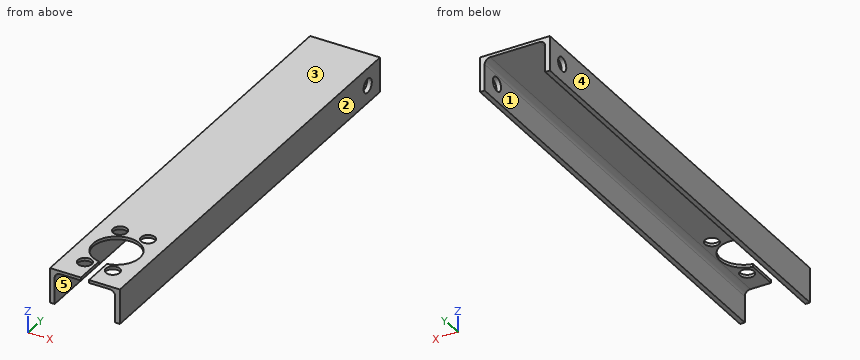
```python
from build123d import *

# Parameters (mm, degrees)
F1_DEPTH = 635
F3_DEPTH = 4.2
F4_R     = 10
F5_DEPTH = 4.2
F6_R     = 10
F7_DEPTH = 100


with BuildPart() as f1:
    # F0 (on Front) → F1 (new body)
    with BuildSketch(Plane.XZ):
        with BuildLine():
            Line((50, 0), (0, 0))
            Line((0, 0), (-50, 0))
            Line((-50, 0), (-50, -50))
            Line((-50, -50), (-43.3, -50))
            Line((-43.3, -50), (-43.3, -12.2))
            ThreePointArc((-43.3, -12.2), (-40.956854, -6.543146), (-35.3, -4.2))
            Line((-35.3, -4.2), (0, -4.2))
            Line((0, -4.2), (35.3, -4.2))
            ThreePointArc((35.3, -4.2), (40.956854, -6.543146), (43.3, -12.2))
            Line((43.3, -12.2), (43.3, -50))
            Line((43.3, -50), (50, -50))
            Line((50, -50), (50, 0))
        make_face()
    extrude(amount=-F1_DEPTH)

    # F2 (on face) → F3 (cut, through all)
    with BuildSketch(Plane.XY):
        with BuildLine():
            Line((5.75, 0), (5.75, 43.997159))
            ThreePointArc((5.75, 43.997159), (0, 110.5), (-5.75, 43.997159))
            Line((-5.75, 43.997159), (-5.75, 0))
            Line((-5.75, 0), (5.75, 0))
        make_face()
    extrude(amount=-F3_DEPTH, mode=Mode.SUBTRACT)

    # F4 (on face) → F5 (cut, through all)
    with BuildSketch(Plane.XY):
        with Locations((-20, 34)):
            Circle(F4_R)
        with Locations((-20, 120)):
            Circle(F4_R)
        with Locations((20, 34)):
            Circle(F4_R)
        with Locations((20, 120)):
            Circle(F4_R)
    extrude(amount=-F5_DEPTH, mode=Mode.SUBTRACT)

    # F6 (on face) → F7 (cut, through all)
    with BuildSketch(Plane(origin=(-50, 0, 0), x_dir=(0, -1, 0), z_dir=(-1, 0, 0))):
        with Locations((-605, -25)):
            Circle(F6_R)
    extrude(amount=-F7_DEPTH, mode=Mode.SUBTRACT)


solid = f1.part
```
Design review of the part built by this model. Coordinates are the model's own, in mm. Face numbers are marked on the shaded views. A direction names the side the tool comes from. Coordinates: 2 decimals unless noted, no trailing zeros. Loops run counter-clockwise (first coordinate to the right, second up) from the corner with the lowest first, then second, coordinate; pieces in that order, holes last. Notation, with made-up numbers: M 40.5,-3.5 L 70.5,-3.5 A21 cw 70.5,26.5 Z; hole C 62,79.5 d8. An arc over 180 degrees is marked long. One line per question, with ' | ' between items.
(1) For pin 1 Ø8 at (x, y) = (13, 103) entering from +Z; pin 2 Ø12 at (x, y) = (33.5, 300.5) entering from +Z; pin 3 Ø21 at (x, y) = (16.5, 169) entering from -Z, all flat-tipped, find the tip position at first contact; note any pin that passes through.
Filled in:
pin 1: passes through | pin 2: stops at z = 0 | pin 3: stops at z = -4.2
(2) We need section B-B (y = 120). Give the boundary of the cut face in (x, z), and give its area (3 significant figures).
Filled in:
outline: M -50,-50 L -43.3,-50 L -43.3,-12.2 A8 cw -35.3,-4.2 L -30,-4.2 L -30,0 L -50,0 Z; M -10,-4.2 L 10,-4.2 L 10,0 L -10,0 Z; M 30,-4.2 L 35.3,-4.2 A8 cw 43.3,-12.2 L 43.3,-50 L 50,-50 L 50,0 L 30,0 Z | area: 893 mm^2
(3) Machinability: for the marked faces 4 and 5, which of the approach directions +Z, -Z, +X, -X, +Y, -Y give a long, thin tool a straight path to every point of the face, cutting with its end or side? Answer none if there is none.
Filled in:
face 4: +Z, -Z, -X, +Y, -Y | face 5: -Z, +Y, -Y
(4) Wall thickness on probe 1 along X at (y, z) = (170.5, -13); probe 2 along Z at (x, y) = (-48, 605); probe 3 along Z at (x, y) = (36, 73): over which ranges is each line inside the solid? List them lowest first.
Filled in:
probe 1: x = -50 to -43.3, 43.3 to 50 | probe 2: z = -50 to -35, -15 to 0 | probe 3: z = -4.23 to 0
(5) Draft analysis for pull direction X (two halves, no side actions). For the marked faces 1, 2 and 3, state which applies: released by +X, released by -X, zero draft, split by the parting line, or undercut.
Filled in:
face 1: undercut | face 2: released by +X | face 3: zero draft
(6) We need section A-A (z = -25). Give the boundary of the cut face in (x, y).
Filled in:
outline: M -50,0 L -43.3,0 L -43.3,595 L -50,595 Z; M -50,615 L -43.3,615 L -43.3,635 L -50,635 Z; M 43.3,0 L 50,0 L 50,595 L 43.3,595 Z; M 43.3,615 L 50,615 L 50,635 L 43.3,635 Z
(7) We need section C-C (x = 20). Give the boundary of the cut face in (y, z).
Filled in:
outline: M 0,-4.2 L 24,-4.2 L 24,0 L 0,0 Z; M 44,-4.2 L 50.13,-4.2 L 50.13,0 L 44,0 Z; M 103.87,-4.2 L 110,-4.2 L 110,0 L 103.87,0 Z; M 130,-4.2 L 635,-4.2 L 635,0 L 130,0 Z
